Part model, mm, in its own coordinate system. A direction names the side the tool comes from. Give positions to 0.01 mm unless a question says otherwise; leave off trailing zeros. Write each loop counter-clockwise with the first axis right and the second up, starting at its lowest first coordinate (ties: lowest second). Pieces come first, ordered by that corner, then holes. Notation, with made-up numbers: (-16.5, -18) - (7.5, -18) arc R23 ccw to (7.5, 14) - close; hole circle Ø7 at (-14.5, 75.5). An arc over 180 degrees is marked (long way). Answer in a Markdown table with one row per item. Add a question column.
1. Band-saw the part on D-D on x = 20. Write the cut outline in (y, z).
2. Pull direction Y, two halves, no side cores. Call faces 4 (the flat face through (39, 19.85, -12)), 5 (the flat face through (72, 12, -15)), 6 (the flat face through (39, 0, -10)), 7 (the flat face through (80, 10, -10)): released by +Y, released by -Y, zero draft, split by the parting line, or undercut.
3. Drop flat-ended pins along their axis: pin 1 Ø4 at (x, z) = (60, -10) entering from -Y; pin 2 Ø5 at (x, y) = (9.5, 10.5) entering from +Z; pin 3 Ø1.5 at (x, z) = (7.5, -10) entering from +Y. Give the stop position or say it passes through.
4. Band-saw the part on C-C on y = 17.75. Write the cut outline in (x, z), plus the area to 3 significant figures.
5. Band-saw the part on B-B on y = 2.25. Write the cut outline in (x, z), plus the area to 3 significant figures.
6. Probe line 1 along X through (y, z) = (5.25, -10); line 2 along Z through (x, y) = (72.5, 18.2); line 3 along Z through (x, y) = (60, 10.75). List the from-to ranges inside material, lowest first.
7. Band-saw the part on A-A on x = 7.5. Write the cut outline in (y, z), plus the area to 3 significant figures.
8. Which spindle directions (+Z, -Z, +X, -X, +Y, -Y) get a long thin tool onto all of the face, cutting with end or side? Do faces 1 (the cylindrical face through (74.807, 7.414, -7.395)), 2 (the cylindrical face through (6.579, 18.29, -10.845)), 3 (the flat face through (0, 10, -10)). Say none if no direction does.
```python
from build123d import *

# Parameters (mm, degrees)
SKETCH1_W                     = 80
SKETCH1_H                     = 20
BOSS_EXTRUDE1_DEPTH           = 19.85
CUT_EXTRUDE1_REACH            = 86.818
SKETCH2_R                     = 3.1
SKETCH3_R                     = 5
CUT_EXTRUDE2_DEPTH            = 15
FILLET1_R                     = 1
CSK_FOR_M6_SFHCS1_D           = 6.6
CSK_FOR_M6_SFHCS1_DEPTH       = 19.85
CSK_FOR_M6_SFHCS1_CSINK_D     = 13.44
CSK_FOR_M6_SFHCS1_CSINK_ANGLE = 90
M3X0_5_TAPPED_HOLE1_REACH     = 86.818
M3X0_5_TAPPED_HOLE1_BORE_R    = 1.25


with BuildPart() as part:
    # Sketch1 → Boss-Extrude1 (new body)
    with BuildSketch(Plane(origin=(0, 0, 0), x_dir=(1, 0, 0), z_dir=(0, 1, 0))):
        with Locations((40, 10)):
            Rectangle(SKETCH1_W, SKETCH1_H)
    extrude(amount=BOSS_EXTRUDE1_DEPTH)

    # Sketch2 → Cut-Extrude1 (cut, up to next)
    with BuildSketch(Plane(origin=(0, 19.85, 0), x_dir=(1, 0, 0), z_dir=(0, 1, 0)), mode=Mode.PRIVATE) as cut_extrude1_sk1:
        with Locations(Location((20, 10, 0), (0, 0, 270))):
            Circle(SKETCH2_R)
    cut_extrude1_tool1 = extrude(cut_extrude1_sk1.sketch, amount=-CUT_EXTRUDE1_REACH, mode=Mode.PRIVATE) & part.part
    # Sketch2 → Cut-Extrude1 (cut, up to next)
    with BuildSketch(Plane(origin=(0, 19.85, 0), x_dir=(1, 0, 0), z_dir=(0, 1, 0)), mode=Mode.PRIVATE) as cut_extrude1_sk2:
        with Locations(Location((60, 10, 0), (0, 0, 270))):
            Circle(SKETCH2_R)
    cut_extrude1_tool2 = extrude(cut_extrude1_sk2.sketch, amount=-CUT_EXTRUDE1_REACH, mode=Mode.PRIVATE) & part.part
    add(cut_extrude1_tool1.solids().sort_by_distance((20, 19.85, -10))[0], mode=Mode.SUBTRACT)
    add(cut_extrude1_tool2.solids().sort_by_distance((60, 19.85, -10))[0], mode=Mode.SUBTRACT)

    # Sketch3 → Cut-Extrude2 (cut)
    with BuildSketch(Plane.XY):
        with Locations((7.5, 11.85)):
            Circle(SKETCH3_R)
        with Locations((72.5, 11.85)):
            Circle(SKETCH3_R)
        with Locations((40, 11.85)):
            Circle(SKETCH3_R)
    extrude(amount=-CUT_EXTRUDE2_DEPTH, mode=Mode.SUBTRACT)

    # Fillet1
    fillet1_edges = [part.edges().sort_by_distance(p)[0] for p in [
        (80, 19.85, -10),
        (40, 19.85, -20),
        (0, 19.85, -10),
        (40, 0, -20),
        (80, 0, -10),
        (40, 0, 0),
        (0, 0, -10),
        (40, 19.85, 0),
        (0, 9.925, -20),
        (80, 9.925, -20),
        (80, 9.925, 0),
        (0, 9.925, 0),
    ]]
    fillet(fillet1_edges, radius=FILLET1_R)

    # CSK for M6 SFHCS1
    with Locations(Plane(origin=(20, 19.85, -10), x_dir=(0, 0, 1), z_dir=(0, 1, 0))):
        with Locations((0, 0), (0, 40)):
            CounterSinkHole(CSK_FOR_M6_SFHCS1_D / 2, CSK_FOR_M6_SFHCS1_CSINK_D / 2, depth=CSK_FOR_M6_SFHCS1_DEPTH, counter_sink_angle=CSK_FOR_M6_SFHCS1_CSINK_ANGLE)

    # M3x0.5 Tapped Hole1 bore → M3x0.5 Tapped Hole1 (cut, up to next)
    with BuildSketch(Plane(origin=(0, 19.85, 0), x_dir=(1, 0, 0), z_dir=(0, 1, 0)), mode=Mode.PRIVATE) as m3x0_5_tapped_hole1_sk1:
        with Locations((7.5, 10)):
            Circle(M3X0_5_TAPPED_HOLE1_BORE_R)
    m3x0_5_tapped_hole1_tool1 = extrude(m3x0_5_tapped_hole1_sk1.sketch, amount=-M3X0_5_TAPPED_HOLE1_REACH, mode=Mode.PRIVATE) & part.part
    # M3x0.5 Tapped Hole1 bore → M3x0.5 Tapped Hole1 (cut, up to next)
    with BuildSketch(Plane(origin=(0, 19.85, 0), x_dir=(1, 0, 0), z_dir=(0, 1, 0)), mode=Mode.PRIVATE) as m3x0_5_tapped_hole1_sk2:
        with Locations((40, 10)):
            Circle(M3X0_5_TAPPED_HOLE1_BORE_R)
    m3x0_5_tapped_hole1_tool2 = extrude(m3x0_5_tapped_hole1_sk2.sketch, amount=-M3X0_5_TAPPED_HOLE1_REACH, mode=Mode.PRIVATE) & part.part
    # M3x0.5 Tapped Hole1 bore → M3x0.5 Tapped Hole1 (cut, up to next)
    with BuildSketch(Plane(origin=(0, 19.85, 0), x_dir=(1, 0, 0), z_dir=(0, 1, 0)), mode=Mode.PRIVATE) as m3x0_5_tapped_hole1_sk3:
        with Locations((72.5, 10)):
            Circle(M3X0_5_TAPPED_HOLE1_BORE_R)
    m3x0_5_tapped_hole1_tool3 = extrude(m3x0_5_tapped_hole1_sk3.sketch, amount=-M3X0_5_TAPPED_HOLE1_REACH, mode=Mode.PRIVATE) & part.part
    add(m3x0_5_tapped_hole1_tool1.solids().sort_by_distance((7.5, 19.85, -10))[0], mode=Mode.SUBTRACT)
    add(m3x0_5_tapped_hole1_tool2.solids().sort_by_distance((40, 19.85, -10))[0], mode=Mode.SUBTRACT)
    add(m3x0_5_tapped_hole1_tool3.solids().sort_by_distance((72.5, 19.85, -10))[0], mode=Mode.SUBTRACT)


solid = part.part
```
Values:
| question | item | result |
|---|---|---|
| 1 | outline | (0, -19) arc R1 ccw to (1, -20) - (18.85, -20) arc R1 ccw to (19.85, -19) - (19.85, -16.72) - (16.43, -13.3) - (0, -13.3) - close; (0, -6.7) - (16.43, -6.7) - (19.85, -3.28) - (19.85, -1) arc R1 ccw to (18.85, 0) - (1, 0) arc R1 ccw to (0, -1) - close |
| 2 | face 4 | released by +Y |
| 2 | face 5 | undercut |
| 2 | face 6 | released by -Y |
| 2 | face 7 | zero draft |
| 3 | pin 1 | passes through |
| 3 | pin 2 | stops at z = -15 |
| 3 | pin 3 | stops at y = 6.91 |
| 4 | outline | (0, -19) arc R1 ccw to (1, -20) - (79, -20) arc R1 ccw to (80, -19) - (80, -1) arc R1 ccw to (79, 0) - (1, 0) arc R1 ccw to (0, -1) - close; hole circle Ø2.5 at (7.5, -10); hole circle Ø9.24 at (20, -10); hole circle Ø2.5 at (40, -10); hole circle Ø9.24 at (60, -10); hole circle Ø2.5 at (72.5, -10) |
| 4 | area | 1,450 mm² |
| 5 | outline | (0, -19) arc R1 ccw to (1, -20) - (79, -20) arc R1 ccw to (80, -19) - (80, -1) arc R1 ccw to (79, 0) - (1, 0) arc R1 ccw to (0, -1) - close; hole circle Ø6.6 at (20, -10); hole circle Ø6.6 at (60, -10) |
| 5 | area | 1,530 mm² |
| 6 | line 1 | x = 0 to 16.7, 23.3 to 56.7, 63.3 to 80 |
| 6 | line 2 | z = -20 to -11.25, -8.75 to 0 |
| 6 | line 3 | z = -20 to -13.3, -6.7 to 0 |
| 7 | outline | (0, -19) arc R1 ccw to (1, -20) - (18.85, -20) arc R1 ccw to (19.85, -19) - (19.85, -11.25) - (16.85, -11.25) - (16.85, -15) - (6.85, -15) - (6.85, 0) - (1, 0) arc R1 ccw to (0, -1) - close; (16.85, -8.75) - (19.85, -8.75) - (19.85, -1) arc R1 ccw to (18.85, 0) - (16.85, 0) - close |
| 7 | area | 239 mm² |
| 8 | face 1 | +Z |
| 8 | face 2 | +Y |
| 8 | face 3 | +Z, -Z, -X, +Y, -Y |
